Answer from the drawing. Dimensions are ordinates in mm from the lowest x, y and z of the part. Give positions to 0.01 mm unless a question says otherwise; leave off trailing zeros. Write each loop counter-clockwise with the first axis right and the second up, starting at its lowest first coordinate (ties: lowest second). Pieces come first, ordered by that corner, then holes. Notation, with made-up numbers: (0.5, 15) - (32.5, 15) arc R13 ccw to (32.5, 26) - close; hole circle Ø3 at (3, -36). An arc over 180 degrees is marked (long way). Write item = value, one per line.
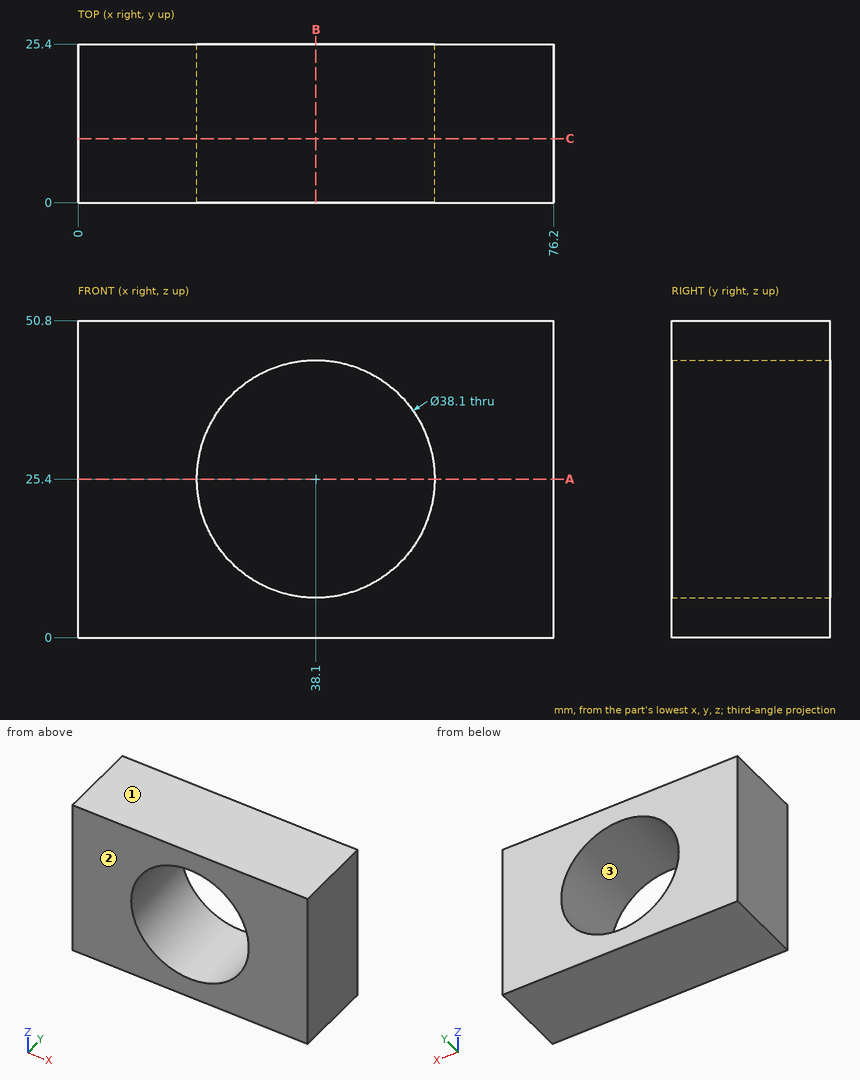
1. Straight lines are drawn through the part: line 1 (Z direction, x = 38.1, y = 18.5); line 2 (X direction, y = 1.5, z = 16); line 3 (Z direction, x = 47, y = 3.75). For each, find the intervals that lie inside material, in ascending order.
Solution:
line_1 = 0 to 6.35, 44.45 to 50.8
line_2 = 0 to 21.53, 54.67 to 76.2
line_3 = 0 to 8.56, 42.24 to 50.8
2. Find section B-B, the plane x = 38.1. Give the vertices of the cut face in (y, z).
Solution:
outline = (0, 0) - (25.4, 0) - (25.4, 6.35) - (0, 6.35) - close; (0, 44.45) - (25.4, 44.45) - (25.4, 50.8) - (0, 50.8) - close
3. Find section A-A, the plane z = 25.4. Give the vertices of the cut face in (x, y).
Solution:
outline = (0, 0) - (19.05, 0) - (19.05, 25.4) - (0, 25.4) - close; (57.15, 0) - (76.2, 0) - (76.2, 25.4) - (57.15, 25.4) - close
4. Find section C-C, the plane y = 10.25. Give the vertices of the cut face in (x, z).
Solution:
outline = (0, 0) - (76.2, 0) - (76.2, 50.8) - (0, 50.8) - close; hole circle Ø38.1 at (38.1, 25.4)
5. For a pull along Z with two mould halves and no side action, classify the marked faces 1, 2 and 3 as pulls with the +Z half, pulls with the -Z half, needs draft (parallel to the pull), parting line crosses it, or undercut.
Solution:
face_1 = pulls with the +Z half
face_2 = needs draft
face_3 = undercut
